Part print with two shaded views. Sizes in mm from the minimum x, y, z corner. A direction names the side the tool comes from. Give positions to 0.01 mm unless a question says otherwise; leave off trailing zeros. Order: outer loops, then holes, each group sorted by start corner. A loop starts at its lowest first (then second) coordinate and runs counter-clockwise, first axis right, second up. Notation, with made-up numbers: M 80,38.5 L 102,38.5 A6 cw 102,45.5 Z; hole C 31.5,70.25 d6. An arc over 180 degrees is marked long. Answer as CSV lines item,"result".
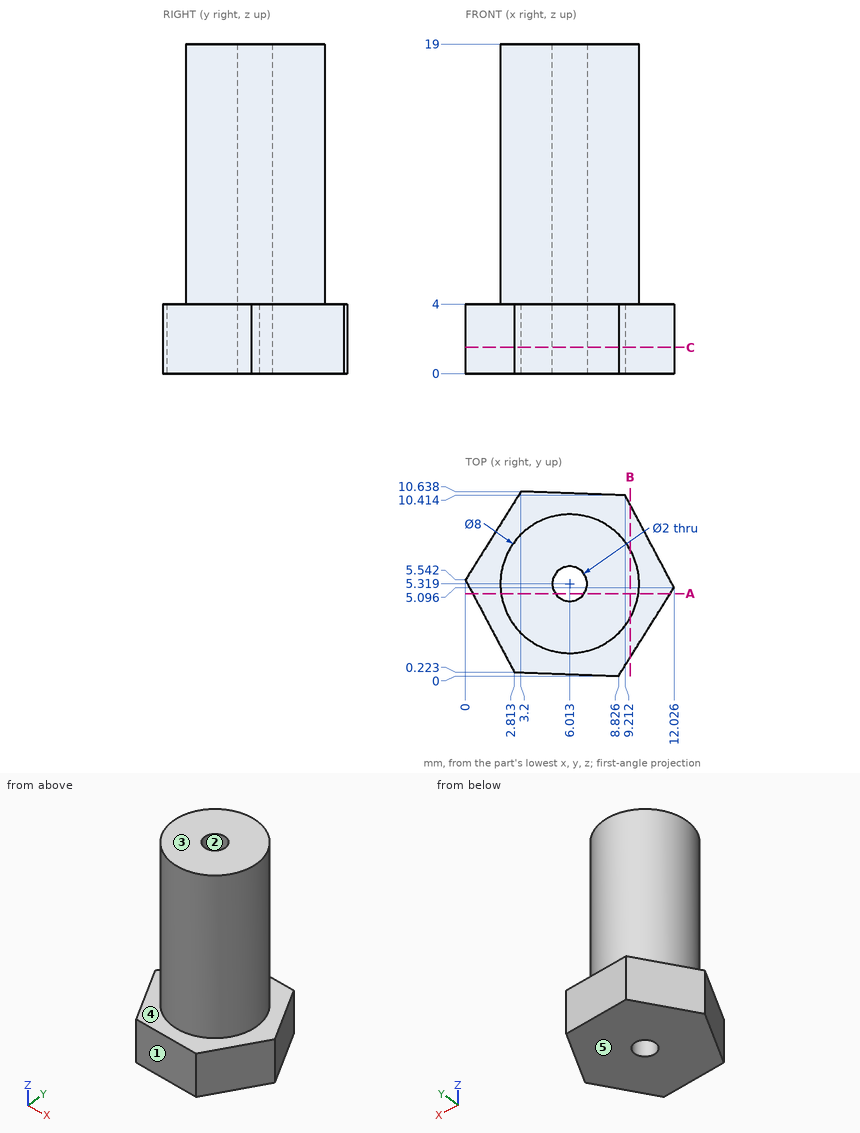
Item 1: Pull direction X, two halves, no side cores. Call the marked faces 1, 2 and 3: released by +X, released by -X, zero draft, split by the parting line, or undercut.
Geometry says:
face 1,"released by -X"
face 2,"undercut"
face 3,"zero draft"
Item 2: 3-axis set-ups, long thin cutter, end or side, ignore diameter. For the marked faces 4 and 5: which of +Z, -Z, +X, -X, +Y, -Y reach the whole face in a straight line?
Geometry says:
face 4,"+Z"
face 5,"-Z, +X, -X, +Y, -Y"
Item 3: Band-saw the part on A-A (y = 4.75). Give the cut face in (x, z) (1 decimal), and give its area (3 significant figures).
Geometry says:
outline,"M 0.4,0 L 5.2,0 L 5.2,19 L 2.1,19 L 2.1,4 L 0.4,4 Z; M 6.8,0 L 11.8,0 L 11.8,4 L 10,4 L 10,19 L 6.8,19 Z"
area,"133 mm2"
Item 4: Band-saw the part on B-B (x = 9.5). Give the cut face in (y, z).
Geometry says:
outline,"M 1.07,0 L 9.87,0 L 9.87,4 L 7.28,4 L 7.28,19 L 3.36,19 L 3.36,4 L 1.07,4 Z"
Item 5: Drop flat-ended pins along their axis: pin 1 (1.6 mm diameter, centred on x = 6.01, y = 5.32, fed in from -Z); pin 2 (6 mm diameter, centred on y = 9, z = 7.5, fed in from +X) (1 decimal). Give the stop position or say it passes through.
Geometry says:
pin 1,"passes through"
pin 2,"stops at x = 10"
Item 6: Probe line 1 along Y through (x, z) = (6, 8.5); line 2 along X through (y, z) = (4.5, 12) (1 decimal); line 3 along Z through (x, y) = (2, 8.25). List the from-to ranges inside material, lowest first. Write a range as from..to.
Geometry says:
line 1,"y = 1.32..4.32, 6.32..9.32"
line 2,"x = 2.1..5.4, 6.6..9.9"
line 3,"z = 0..4"
Item 7: Band-saw the part on C-C (z = 1.5). Give the cut face in (x, y) (1 decimal).
Geometry says:
outline,"M 0,5.5 L 2.8,0.2 L 8.8,0 L 12,5.1 L 9.2,10.4 L 3.2,10.6 Z; hole C 6,5.3 d2"
